Part model, mm, in its own coordinate system. Face numbers are marked on the shaded views. A direction names the side the tool comes from. Give positions to 0.01 mm unless a question says otherwise; leave off trailing zeros. Write each loop counter-clockwise with the first axis right and the second up, starting at its lowest first coordinate (ties: lowest second). Pieces come first, ordered by that corner, then holes. Notation, with made-up numbers: M 13.25,20.25 L 36.25,20.25 A18 ccw 36.25,40.25 Z; hole C -25.5,5 d3. An arc over 180 degrees is marked long. Answer as CSV lines item,"result". Start each with the question number.
Item 1: Pin check, flat tips, straight feed: pin 1 (1.5 mm diameter, centred on y = -13.5, z = -3, fed in from +X); pin 2 (5 mm diameter, centred on x = -14.5, z = 6, fed in from -Y); pin 3 (3 mm diameter, centred on y = 0.5, z = 1.5, fed in from +X); pin 4 (3.5 mm diameter, centred on y = 0, z = 0, fed in from +X). Stop position of each tip, or through.
Item 2: Band-saw the part on B-B, the plane y = 0. List the corners of the cut face in (x, z) (3 decimals).
Item 3: Band-saw the part on A-A, the plane y = -27.5. List the corners of the cut face in (x, z), then the cut area to 4 significant figures.
Item 4: 3-axis set-ups, long thin cutter, end or side, ignore diameter. For the marked faces 1, 2 and 3: which of +Z, -Z, +X, -X, +Y, -Y reach the whole face in a straight line?
Item 5: Band-saw the part on C-C, the plane z = 0. Count the separate pieces of the cut face and the enclosed holes in it, then the cut area to 3 significant figures.
Item 6: Two-plate mould, pull along Z, no slides. Class the marked faces 4, 5, 6 and 7: +Z half, -Z half, draft (parallel to the pull), parting line (faces both ways), or undercut.
Item 7: Wall check: L1, parallel to Z at x = -7.4, y = -27.5; L2, parallel to X at y = 4, z = -0.25 (3 decimals); L3, parallel to Y at x = -14.4, z = 0. Give the ranges that are in metal, low to high. Write a range as from..to.
from build123d import *

# Parameters (mm, degrees)
FILLET1_R               = 7
M5_CLEARANCE_HOLE1_D    = 5.5
CUT_EXTRUDE1_DEPTH      = 37.52886072966826
CUT_EXTRUDE1_DEPTH_BACK = 37.52886072966826
SKETCH3_R               = 2.4999999999999996


with BuildPart() as part:
    # Sweep1: sweep along a path in Sketch1
    with BuildLine(Plane.XY) as sweep1_path:
        Line((-14.2875, 7.5), (-14.2875, -7.5))
        ThreePointArc((-14.2875, -7.5), (-8.903716825795872, -12.735560659438995), (-7.000000000000001, -20))
        Line((-7.000000000000001, -20), (-6.999999999999999, -35))
    # Sketch2 → Sweep1 (sweep)
    with BuildSketch(Plane(origin=(0, 0, 0), x_dir=(1, 0, 0), z_dir=(0, 1, 0))):
        Polygon((-12.699999999999996, -7.499999999999996), (-15.874999999999996, -7.499999999999996), (-15.874999999999996, 7.500000000000004), (-12.699999999999996, 7.500000000000005), align=None)
    sweep(path=sweep1_path.line, transition=Transition.RIGHT)

    # Fillet1
    fillet1_edges = [part.edges().sort_by_distance(p)[0] for p in [
        (-15.874999999999996, -8.441785890670294, -1.599e-14),
        (-12.699999999999996, -6.5917812273426035, -7.11e-15),
    ]]
    fillet(fillet1_edges, radius=FILLET1_R)

    # M5 Clearance Hole1 (through all)
    with Locations(Plane.ZY.offset(15.874999999999996)):
        with Locations((0, 0)):
            Hole(M5_CLEARANCE_HOLE1_D / 2)

    # Sketch3 → Cut-Extrude1 (cut, two sides: drawn at the far end of the back side and taken through both)
    with BuildSketch(Plane.ZY.offset(8.587500000000007).offset(-CUT_EXTRUDE1_DEPTH_BACK)):
        with Locations(Location((0, -27.500000000000004, 0), (0, 0, 270))):
            Circle(SKETCH3_R)
    extrude(amount=CUT_EXTRUDE1_DEPTH + CUT_EXTRUDE1_DEPTH_BACK, mode=Mode.SUBTRACT)


solid = part.part
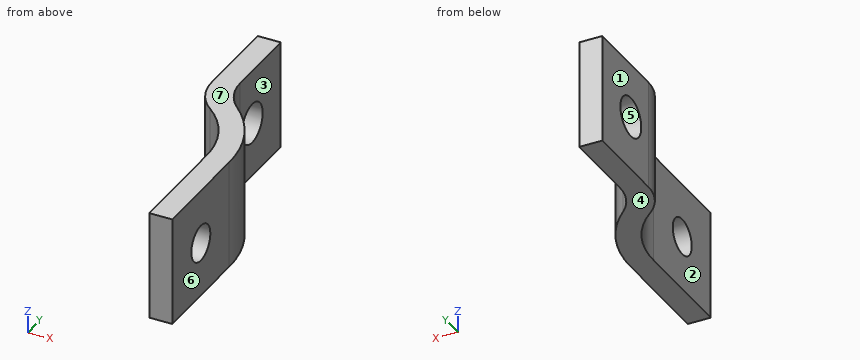
Output:
1,pin 1,"x = -6.43"
1,pin 2,"y = -11.24"
1,pin 3,"x = -12.7"
1,pin 4,"through"
2,outline,"M -15.875,-7.5 L -12.7,-7.5 L -12.7,-2.75 L -15.875,-2.75 Z; M -15.875,2.75 L -12.7,2.75 L -12.7,7.5 L -15.875,7.5 Z"
3,outline,"M -8.59,-7.5 L -5.41,-7.5 L -5.41,-2.5 L -8.59,-2.5 Z; M -8.59,2.5 L -5.41,2.5 L -5.41,7.5 L -8.59,7.5 Z"
3,area,"31.75 mm²"
4,face 1,"+Z, -Z, -X, +Y, -Y"
4,face 2,"+Z, -Z, -X, -Y"
4,face 3,"+Z, -Z, +X, +Y"
5,separate pieces,"3"
5,enclosed holes,"0"
5,area,"110 mm²"
6,face 4,"-Z half"
6,face 5,"undercut"
6,face 6,"draft"
6,face 7,"+Z half"
7,L1,"-7.5..-2.5, 2.5..7.5"
7,L2,"-15.875..-12.7"
7,L3,"-8.92..-2.75, 2.75..7.5"
